Work out the finished part from the listing and answer in its coordinate system (mm). Face numbers are marked on the shaded views. A direction names the side the tool comes from. Round coordinates to 2 decimals unless told otherwise and drop trailing zeros. Order: outer loops, then holes, each group sorted by start corner. A loop starts at its lowest first (then second) coordinate and runs counter-clockwise, first axis right, second up. Notation, with made-up numbers: (-36.75, -5) - (-18.75, -5) arc R19 ccw to (-18.75, 12) - close; hole circle Ø10 at (89.5, -11). An arc over 180 degrees is marked (long way). Answer in a Markdown table with one row per item.
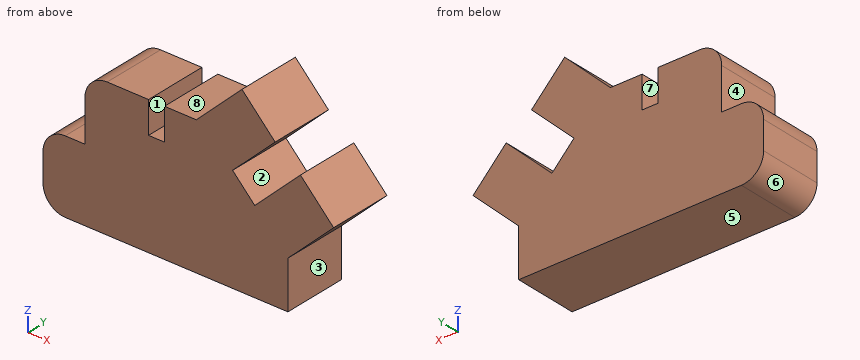
from build123d import *

# Parameters (mm, degrees)
F1_DEPTH = 508


with BuildPart() as f1:
    # F0 (on Front) → F1 (new body)
    with BuildSketch(Plane.XZ):
        with BuildLine():
            Line((-940.237215, 192.609879), (-940.237215, -30.321289))
            ThreePointArc((-940.237215, -30.321289), (-888.160801, -156.044874), (-762.437215, -208.121289))
            Line((-762.437215, -208.121289), (1015.562785, -208.121289))
            Line((1015.562785, -208.121289), (1015.562785, 172.878711))
            Line((1015.562785, 172.878711), (1380.703211, 526.059216))
            Line((1380.703211, 526.059216), (1115.817833, 799.914536))
            Line((1115.817833, 799.914536), (750.677406, 446.734031))
            Line((750.677406, 446.734031), (574.087154, 629.304244))
            Line((574.087154, 629.304244), (913.639785, 957.735064))
            Line((913.639785, 957.735064), (648.754406, 1231.590384))
            Line((648.754406, 1231.590384), (283.613979, 878.409879))
            Line((283.613979, 878.409879), (29.613979, 878.409879))
            Line((29.613979, 878.409879), (29.613979, 624.409879))
            Line((29.613979, 624.409879), (-97.386021, 624.409879))
            Line((-97.386021, 624.409879), (-97.386021, 878.409879))
            Line((-97.386021, 878.409879), (-427.586021, 878.409879))
            ThreePointArc((-427.586021, 878.409879), (-553.309606, 826.333464), (-605.386021, 700.609879))
            Line((-605.386021, 700.609879), (-605.386021, 370.409879))
            Line((-605.386021, 370.409879), (-762.437215, 370.409879))
            ThreePointArc((-762.437215, 370.409879), (-888.160801, 318.333464), (-940.237215, 192.609879))
        make_face()
    extrude(amount=F1_DEPTH)


solid = f1.part
1) Find section B-B, the plane y = -333. Give the vertices of the cut face in (x, z).
Filled in:
| item | result |
|---|---|
| outline | (-940.24, -30.32) arc R177.8 ccw to (-762.44, -208.12) - (1015.56, -208.12) - (1015.56, 172.88) - (1380.7, 526.06) - (1115.82, 799.91) - (750.68, 446.73) - (574.09, 629.3) - (913.64, 957.74) - (648.75, 1231.59) - (283.61, 878.41) - (29.61, 878.41) - (29.61, 624.41) - (-97.39, 624.41) - (-97.39, 878.41) - (-427.59, 878.41) arc R177.8 ccw to (-605.39, 700.61) - (-605.39, 370.41) - (-762.44, 370.41) arc R177.8 ccw to (-940.24, 192.61) - close |
2) Find section A-A, the plane z = 731. Give the vertices of the cut face in (x, y), then the cut area to 3 significant figures.
Filled in:
| item | result |
|---|---|
| outline | (-602.77, -508) - (-97.39, -508) - (-97.39, 0) - (-602.77, 0) - close; (29.61, -508) - (679.23, -508) - (679.23, 0) - (29.61, 0) - close; (1044.57, -508) - (1182.48, -508) - (1182.48, 0) - (1044.57, 0) - close |
| area | 657,000 mm^2 |
3) Each of these flat-tipped pins is pushed along its axis until it touches: pin 1 (8 mm diameter, centred on y = -268, z = 723.5, fed in from -X); pin 2 (4 mm diameter, centred on x = -186, y = -236.5, fed in from +Z); pin 3 (10 mm diameter, centred on x = -463, y = -196.5, fed in from +Z). Where does it stop, or does it pass through?
Filled in:
| item | result |
|---|---|
| pin 1 | stops at x = -604.38 |
| pin 2 | stops at z = 878.41 |
| pin 3 | stops at z = 875.79 |
4) Find section D-D, the plane x = -144.5. Give the vertices of the cut face in (y, z), then the cut area to 3 significant figures.
Filled in:
| item | result |
|---|---|
| outline | (-508, -208.12) - (0, -208.12) - (0, 878.41) - (-508, 878.41) - close |
| area | 552,000 mm^2 |
5) Find section C-C, the plane x = 692.5. Give the vertices of the cut face in (y, z).
Filled in:
| item | result |
|---|---|
| outline | (-508, -208.12) - (0, -208.12) - (0, 506.88) - (-508, 506.88) - close; (-508, 743.84) - (0, 743.84) - (0, 1186.36) - (-508, 1186.36) - close |
6) The mould has two halves that part along X. Classify the marked faces 6, 7 and 8: released by +X, released by -X, zero draft, split by the parting line, or undercut.
Filled in:
| item | result |
|---|---|
| face 6 | released by -X |
| face 7 | undercut |
| face 8 | zero draft |
7) Which of the six approach directions +Z, -Z, +X, -X, +Y, -Y give full straight-line access (tool end or side, diameter ignored) to the marked faces 1, 2, 3, 4 and 5?
Filled in:
| item | result |
|---|---|
| face 1 | +Z, +Y, -Y |
| face 2 | +Y, -Y |
| face 3 | -Z, +X, +Y, -Y |
| face 4 | +Z, -X, +Y, -Y |
| face 5 | -Z, +X, -X, +Y, -Y |
8) Find the intervals of material crossed by probe 1 along X at (y, z) = (-264.5, 650.5); probe 2 along Z at (x, y) = (161, -24); probe 3 along Z at (x, y) = (-772, -266.5), in increasing order. Write a range as from..to.
Filled in:
| item | result |
|---|---|
| probe 1 | x = -605.39..-97.39, 29.61..596, 961.34..1260.34 |
| probe 2 | z = -208.12..878.41 |
| probe 3 | z = -207.86..370.15 |
